Build history of the part. All positions in model axes, mm. A direction names the side the tool comes from. Give positions to 0.01 mm unless a question says otherwise; leave off trailing zeros. Loops run counter-clockwise (first coordinate to the right, second up) from the corner with the lowest first, then second, coordinate; pieces in that order, holes last. Notation, with made-up numbers: (-7, 21) -> (0, 21) arc R16 cw to (0, 38) -> close; hole circle Ø9 at (41, -33). An arc over 180 degrees is marked (long way). Answer as a JSON object with one key per item and string values. Group by question number.
Q1. Drop flat-ended pins along their axis: pin 1 (15 mm diameter, centred on x = 47, y = 31, fed in from +Z); pin 2 (5 mm diameter, centred on x = -71.5, y = 9, fed in from +Z). Give the stop position or say it passes through.
Q2. Band-saw the part on C-C, the plane x = 37. Write the cut outline in (y, z).
Q3. Two-plate mould, pull along X, no slides. Class faces 1 (the flat face through (125, 35, -15)), 2 (the flat face through (-1, 60, -15)), 3 (the flat face through (120, 35, 0)): pulls with the +X half, pulls with the -X half, needs draft (parallel to the pull), parting line crosses it, or undercut.
Q4. Band-saw the part on D-D, the plane y = 52. Write the cut outline in (x, z).
Q5. Band-saw the part on B-B, the plane y = 35. Write the cut outline in (x, z), plus the area to 3 significant figures.
Q6. Tool access for faces 4 (the flat face through (115, 35, -5)), 5 (the cylindrical face through (-0.745, 39.957, -24.93)), 6 (the flat face through (102, 35, -15)): list every direction of +Z, -Z, +X, -X, +Y, -Y with a clear straight run to the whole face (end or side of a thin tool).
Q7. Band-saw the part on A-A, the plane z = -3. Write the cut outline in (x, y), plus the area to 3 significant figures.
Q8. Wall check: probe 1 along Y at (x, z) = (-73.5, -11); probe 2 along X at (y, z) = (21, -3); probe 3 along Z at (x, y) = (13, 26). Give the ranges that are in metal, low to high. Write a range as from..to.
from build123d import *

# Parameters (mm, degrees)
SKETCH1_R           = 5
BOSS_EXTRUDE1_DEPTH = 70
SKETCH3_W           = 50
SKETCH3_H           = 30
CUT_EXTRUDE1_DEPTH  = 266.171642526
SKETCH6_W           = 230
SKETCH6_H           = 50
CUT_EXTRUDE2_DEPTH  = 20
SKETCH7_R           = 5
CUT_EXTRUDE3_DEPTH  = 148.244694302
SKETCH8_W           = 34.830665203
SKETCH8_H           = 70
CUT_EXTRUDE4_DEPTH  = 266.171642526
SKETCH9_W           = 230
SKETCH9_H           = 10
CUT_EXTRUDE5_DEPTH  = 147.372811683
SKETCH10_W          = 13
SKETCH10_H          = 50
BOSS_EXTRUDE4_DEPTH = 10


with BuildPart() as part:
    # Sketch1 → Boss-Extrude1 (new body)
    with BuildSketch(Plane(origin=(0, 0, 0), x_dir=(1, 0, 0), z_dir=(0, 1, 0))):
        with BuildLine():
            Line((-125, 0), (125, 0))
            Line((125, 0), (125, 30))
            Line((125, 30), (119.5, 30))
            Line((119.5, 30), (119.5, 42))
            ThreePointArc((119.5, 42), (107.5, 54), (95.5, 42))
            Line((95.5, 42), (95.5, 30))
            Line((95.5, 30), (-95.5, 30))
            Line((-95.5, 30), (-95.5, 42))
            ThreePointArc((-95.5, 42), (-107.5, 54), (-119.5, 42))
            Line((-119.5, 42), (-119.5, 30))
            Line((-119.5, 30), (-125, 30))
            Line((-125, 30), (-125, 0))
        make_face()
        with Locations(Location((107.5, 42, 0), (0, 0, 270))):
            Circle(SKETCH1_R, mode=Mode.SUBTRACT)
        with Locations(Location((-107.5, 42, 0), (0, 0, 270))):
            Circle(SKETCH1_R, mode=Mode.SUBTRACT)
    extrude(amount=BOSS_EXTRUDE1_DEPTH)

    # Sketch3 → Cut-Extrude1 (cut, through all)
    with BuildSketch(Plane.ZY.offset(125)):
        with Locations((-55, 15)):
            Rectangle(SKETCH3_W, SKETCH3_H)
    extrude(amount=-CUT_EXTRUDE1_DEPTH, mode=Mode.SUBTRACT)

    # Sketch6 → Cut-Extrude2 (cut)
    with BuildSketch(Plane.XY):
        with Locations((0, 35)):
            Rectangle(SKETCH6_W, SKETCH6_H)
    extrude(amount=-CUT_EXTRUDE2_DEPTH, mode=Mode.SUBTRACT)

    # Sketch7 → Cut-Extrude3 (cut, through all)
    with BuildSketch(Plane.XY.offset(-20)):
        with Locations((-0.094237072, 35)):
            Circle(SKETCH7_R)
    extrude(amount=-CUT_EXTRUDE3_DEPTH, mode=Mode.SUBTRACT)

    # Sketch8 → Cut-Extrude4 (cut, through all)
    with BuildSketch(Plane(origin=(125, 0, 0), x_dir=(0, 0, -1), z_dir=(1, 0, 0))):
        with Locations((47.415332602, 35)):
            Rectangle(SKETCH8_W, SKETCH8_H)
    extrude(amount=-CUT_EXTRUDE4_DEPTH, mode=Mode.SUBTRACT)

    # Sketch9 → Cut-Extrude5 (cut, through all)
    with BuildSketch(Plane(origin=(0, 70, 0), x_dir=(1, 0, 0), z_dir=(0, 1, 0))):
        with Locations((0, 5)):
            Rectangle(SKETCH9_W, SKETCH9_H)
    extrude(amount=-CUT_EXTRUDE5_DEPTH, mode=Mode.SUBTRACT)

    # Sketch10 → Boss-Extrude4 (add)
    with BuildSketch(Plane.XY.offset(-20)):
        with Locations((-108.5, 35)):
            Rectangle(SKETCH10_W, SKETCH10_H)
        with Locations((108.5, 35)):
            Rectangle(SKETCH10_W, SKETCH10_H)
    extrude(amount=BOSS_EXTRUDE4_DEPTH)


solid = part.part
Worked answers:
{
 "1": {"pin 1": "z = -20", "pin 2": "z = -10"},
 "2": {"outline": "(0, -30) -> (70, -30) -> (70, -10) -> (60, -10) -> (60, -20) -> (10, -20) -> (10, -10) -> (0, -10) -> close"},
 "3": {"face 1": "pulls with the +X half", "face 2": "undercut", "face 3": "needs draft"},
 "4": {"outline": "(-125, -30) -> (125, -30) -> (125, 0) -> (115, 0) -> (115, -10) -> (102, -10) -> (102, -20) -> (-102, -20) -> (-102, -10) -> (-115, -10) -> (-115, 0) -> (-125, 0) -> close"},
 "5": {"outline": "(-125, -30) -> (-5.09, -30) -> (-5.09, -20) -> (-102, -20) -> (-102, -10) -> (-115, -10) -> (-115, 0) -> (-125, 0) -> close; (4.91, -30) -> (125, -30) -> (125, 0) -> (115, 0) -> (115, -10) -> (102, -10) -> (102, -20) -> (4.91, -20) -> close", "area": "3,060 mm2"},
 "6": {"face 4": "+Z, +Y, -Y", "face 5": "+Z, -Z", "face 6": "+Z"},
 "7": {"outline": "(-125, 0) -> (-115, 0) -> (-115, 70) -> (-125, 70) -> close; (115, 0) -> (125, 0) -> (125, 70) -> (115, 70) -> close", "area": "1,400 mm2"},
 "8": {"probe 1": "0..10, 60..70", "probe 2": "-125..-115, 115..125", "probe 3": "-30..-20"}
}
